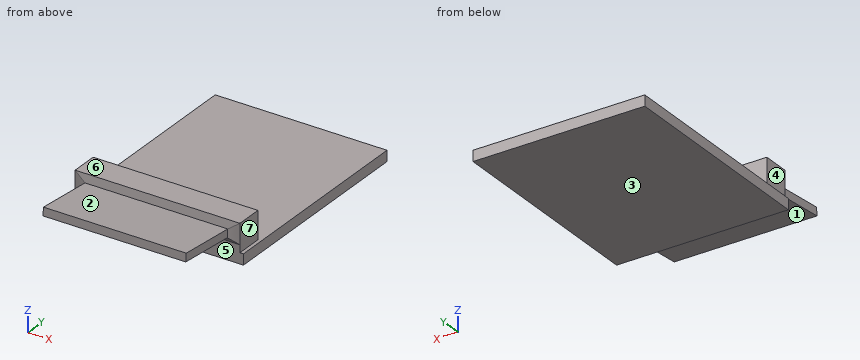
```python
from build123d import *

# Parameters (mm, degrees)
F0_W      = 16
F0_H      = 20
F1_DEPTH  = 1
F2_W      = 15.35
F2_H      = 2.5
F3_DEPTH  = 2.6
F7_W      = 13.3
F7_H      = 0.75
F8_DEPTH  = 5.8
F4_W      = 15.35
F4_H      = 1.9
F8_FACE_W = 13.3
F8_FACE_H = 0.75


with BuildPart() as f1:
    # F0 (on Top) → F1 (new body)
    with BuildSketch(Plane.XY):
        Rectangle(F0_W, F0_H)
    extrude(amount=F1_DEPTH)

    # F2 (on face) → F3 (join)
    with BuildSketch(Plane.XY.offset(1)):
        with Locations((0, -8.75)):
            Rectangle(F2_W, F2_H)
    extrude(amount=F3_DEPTH)



with BuildPart() as f8:
    # F7 (on face) → F8 (new body)
    with BuildSketch(Plane(origin=(0, -10.3362249547, 0.9043025072), x_dir=(-1, 0, 0), z_dir=(0, 0.9961946981, -0.0871557427))):
        with Locations((0, 1.5897434857)):
            Rectangle(F7_W, F7_H)
    extrude(amount=-F8_DEPTH)


with BuildPart() as f1_1:
    add(f1.part)

    add(f8.part)  # F9 merges F8
    # F4 (on face) → F9 section 0
    with BuildSketch(Plane.XZ.offset(10)):
        with Locations((0, 2.65)):
            Rectangle(F4_W, F4_H)
    # F8_face (on face) → F9 section 1
    with BuildSketch(Plane(origin=(0, -10.1976696804, 2.4879965389), x_dir=(-1, 0, 0), z_dir=(0, 0.9961946981, -0.0871557427))):
        Rectangle(F8_FACE_W, F8_FACE_H)
    loft()


solid = f1_1.part
```
Check sheet for the modelled part. Datum: model origin and axes. Units: mm. Face numbers are marked on the shaded views. A direction names the side the tool comes from. Give positions to 0.01 mm unless a question says otherwise; leave off trailing zeros. Write each loop counter-clockwise with the first axis right and the second up, starting at its lowest first coordinate (ties: lowest second). Pieces come first, ordered by that corner, then holes.
Item 1: Cross-section at B-B (z = 0.7). Enter the section's corners in (x, y).
Item 2: Cross-section at C-C (y = 0.5). Enter the section's corners in (x, z), and give its area (3 significant figures).
Item 3: Gauge pin test, flat ends, axial feed: pin 1 (0.5 mm diameter, centred on x = -2.5, z = 1, fed in from -Y); pin 2 (1.4 mm diameter, centred on y = -12.5, z = 3, fed in from -X); pin 3 (8 mm diameter, centred on x = -0.5, y = 2.5, fed in from +Z); pin 4 (8 mm diameter, centred on x = -2.5, y = 2, fed in from -Z). Record the tip position at first contact, or that the pin passes through.
Item 4: Draft check along Y on the marked faces 1, 2 and 3. Enter one of: released by +Y, released by -Y, zero draft, split by the parting line, or undercut.
Item 5: Access from +Z, -Z, +X, -X, +Y, -Y to the whole of each face (thin tool, end or side, straight path). Record for the marked faces 4, 5, 6 and 7.
Item 6: Scan lines: L1, parallel to Z at x = -2.75, y = 3.5; L2, parallel to Y at x = -7.25, z = 0.8; L3, parallel to Z at x = 0.25, y = -12. Record each from-to range of solid material in increasing order.
Item 7: Cross-section at A-A (y = -8.5). Enter the section's corners in (x, z) (3 decimals).
Report:
1. outline: (-8, -10) - (8, -10) - (8, 10) - (-8, 10) - close
2. outline: (-8, 0) - (8, 0) - (8, 1) - (-8, 1) - close
2. area: 16.0 mm2
3. pin 1: stops at y = -10
3. pin 2: stops at x = -6.65
3. pin 3: stops at z = 1
3. pin 4: stops at z = 0
4. face 1: released by -Y
4. face 2: undercut
4. face 3: zero draft
5. face 4: +Z, -X, +Y, -Y
5. face 5: -Z, +X, -X, -Y
5. face 6: +Z, +X, -X, +Y, -Y
5. face 7: +Z, +X, +Y, -Y
6. L1: z = 0 to 1
6. L2: y = -10 to 10
6. L3: z = 2.27 to 3.02
7. outline: (-8, 0) - (8, 0) - (8, 1) - (7.675, 1) - (7.675, 3.6) - (-7.675, 3.6) - (-7.675, 1) - (-8, 1) - close
